The listing builds one solid part. Answer for the finished solid, in the listing's coordinates (mm). Coordinates: 2 decimals unless noted, no trailing zeros. Order: outer loops, then holes, each group sorted by start corner. A loop starts at its lowest first (then second) coordinate and runs counter-clockwise, first axis right, second up.
from build123d import *

# Parameters (mm, degrees)
ESQUISSE1_R        = 1.5
BOSS_EXTRU_1_DEPTH = 2.4
CHANFREIN1_SIZE    = 0.25


with BuildPart() as part:
    # Esquisse1 → Boss.-Extru.1 (new body)
    with BuildSketch(Plane.XY):
        Polygon((0, -3), (2.598076211, -1.5), (2.598076211, 1.5), (0, 3), (-2.598076211, 1.5), (-2.598076211, -1.5), align=None)
        Circle(ESQUISSE1_R, mode=Mode.SUBTRACT)
    extrude(amount=BOSS_EXTRU_1_DEPTH)

    # Chanfrein1
    chanfrein1_edges = [part.edges().sort_by_distance(p)[0] for p in [
        (2.598076211, 0, 2.4),
        (1.299038106, 2.25, 2.4),
        (-1.299038106, 2.25, 2.4),
        (-2.598076211, 0, 2.4),
        (-1.299038106, -2.25, 2.4),
        (1.299038106, -2.25, 2.4),
    ]]
    chamfer(chanfrein1_edges, length=CHANFREIN1_SIZE)


solid = part.part
1) This flat-tipped pin is pushed along its axis until it touches: P1, Ø1, axis at x = 2, z = 2, coming from the +Y side. Where does it stop, or does it pass through?
2) Section B-B (x = 0.35) is taken. Give the vertices of the cut face in (y, z), then the cut area to 3 significant figures.
3) Section C-C (z = 0.8) is taken. Give the vertices of the cut face in (x, y).
4) Section D-D (y = -2.25) is taken. Give the vertices of the cut face in (x, z).
5) Section A-A (y = 0) is taken. Give the vertices of the cut face in (x, z).
6) Determine the mould class of faces 1 (the face through (2, 0, 2.4)), 2 (the face through (-1.5, 0.07, 1.18)), 3 (the face through (2.598, 0, 1)) for opening direction X: released by +X, released by -X, zero draft, split by the parting line, or undercut.
7) Consider L1, parallel to X at y = -0.5, z = 0.1; L2, parallel to Y at x = -1.05, z = 0.7; L3, parallel to Y at x = -0.65, z = 1.1. Determine where each line is inside the solid, lowest interval first.
Filled sheet:
1. P1: stops at y = 2.13
2. outline: (-2.8, 0) - (-1.46, 0) - (-1.46, 2.4) - (-2.51, 2.4) - (-2.8, 2.15) - close; (1.46, 0) - (2.8, 0) - (2.8, 2.15) - (2.51, 2.4) - (1.46, 2.4) - close
2. area: 6.36 mm2
3. outline: (-2.6, -1.5) - (0, -3) - (2.6, -1.5) - (2.6, 1.5) - (0, 3) - (-2.6, 1.5) - close; hole circle Ø3 at (0, 0)
4. outline: (-1.3, 0) - (1.3, 0) - (1.3, 2.15) - (0.8, 2.4) - (-0.8, 2.4) - (-1.3, 2.15) - close
5. outline: (-2.6, 0) - (-1.5, 0) - (-1.5, 2.4) - (-2.35, 2.4) - (-2.6, 2.15) - close; (1.5, 0) - (2.6, 0) - (2.6, 2.15) - (2.35, 2.4) - (1.5, 2.4) - close
6. face 1: zero draft
6. face 2: undercut
6. face 3: released by +X
7. L1: x = -2.6 to -1.41, 1.41 to 2.6
7. L2: y = -2.39 to -1.07, 1.07 to 2.39
7. L3: y = -2.62 to -1.35, 1.35 to 2.62
